Model file for the job. Use its own axes, mm. A direction names the side the tool comes from. Round coordinates to 2 decimals unless told otherwise and drop trailing zeros. Loops run counter-clockwise (first coordinate to the right, second up) from the corner with the lowest first, then second, coordinate; pieces in that order, holes last. Notation, with made-up numbers: M -24.5,31.5 L 13.5,31.5 A17 cw 13.5,38.5 Z; hole C 69.25,-5 d4. An arc over 180 degrees is marked long. Use a Markdown table: item, result. Add a question column.
Q1. Pin check, flat tips, straight feed: pin 1 (1.5 mm diameter, centred on x = 49.5, y = 1, fed in from +Z); pin 2 (1 mm diameter, centred on y = 1.5, z = 16, fed in from +X); pin 3 (3.5 mm diameter, centred on x = 12.5, z = 15, fed in from +Y). Stop position of each tip, or through.
Q2. Cut at C-C (x = 61). Give the cut face in (y, z).
Q3. Mould opens along Z. For faces 1 (the face through (47, 1, 7.5)), 2 (the face through (12.59, 1.48, 17.1)), 3 (the face through (-1, 3, 4)), 4 (the face through (-1, 1, -7.5)) say: +Z half, -Z half, draft (parallel to the pull), parting line (faces both ways), or undercut.
Q4. Probe line 1 (X direction, y = 1.4, z = 0); line 2 (X direction, y = 1.9, z = 15.25); line 3 (Z direction, x = 58, y = 2.1). List the from-to ranges inside material, lowest first. Write a range as from..to.
Q5. Cut at B-B (x = 42.5). Give the cut face in (y, z).
Q6. Tool access for faces 5 (the face through (-46, 1, 7.5)), 6 (the face through (-43.92, 1.48, 0.74)): list every direction of +Z, -Z, +X, -X, +Y, -Y with a clear straight run to the whole face (end or side of a thin tool).
Q7. Cut at A-A (y = 0.5). Give the cut face in (x, z).
Q8. Cut at D-D (z = 10.5). Give the cut face in (x, y), plus the area to 3 significant figures.
from build123d import *

# Parameters (mm, degrees)
SKETCH_1_R          = 1.6
SKETCH_1_R_2        = 2.1
EXTRUDE_1_DEPTH     = 3
SKETCH_3_W          = 40
SKETCH_3_H          = 3
EXTRUDE_3_DEPTH     = 15
SKETCH_2_R          = 2.1
CUT_EXTRUDE_1_DEPTH = 76.970388968
FILLET_START        = -1
FILLET_2_DEPTH      = 5
FILLET_2_2_DEPTH    = 3


with BuildPart() as part:
    # 草图1 → 凸台-拉伸1 (new body)
    with BuildSketch(Plane(origin=(0, 0, 0), x_dir=(1, 0, 0), z_dir=(0, 1, 0))):
        with BuildLine():
            Line((-65, 7.5), (65, 7.5))
            ThreePointArc((65, 7.5), (72.5, 0), (65, -7.5))
            Line((65, -7.5), (-65, -7.5))
            ThreePointArc((-65, -7.5), (-72.5, 0), (-65, 7.5))
        make_face()
        with Locations(Location((-42.5, 0, 0), (0, 0, 270))):
            Circle(SKETCH_1_R, mode=Mode.SUBTRACT)
        with Locations(Location((-65, 0, 0), (0, 0, 270))):
            Circle(SKETCH_1_R_2, mode=Mode.SUBTRACT)
        with Locations(Location((65, 0, 0), (0, 0, 270))):
            Circle(SKETCH_1_R_2, mode=Mode.SUBTRACT)
        with Locations(Location((42.5, 0, 0), (0, 0, 270))):
            Circle(SKETCH_1_R, mode=Mode.SUBTRACT)
    extrude(amount=EXTRUDE_1_DEPTH)

    # 草图3 → 凸台-拉伸3 (add)
    with BuildSketch(Plane.XY.offset(7.5)):
        with Locations((0, 1.5)):
            Rectangle(SKETCH_3_W, SKETCH_3_H)
    extrude(amount=EXTRUDE_3_DEPTH)

    # 草图2 → 切除-拉伸1 (cut, through all)
    with BuildSketch(Plane.XZ):
        with Locations(Location((-12.5, 15, 0), (0, 0, 270))):
            Circle(SKETCH_2_R)
        with Locations(Location((12.5, 15, 0), (0, 0, 270))):
            Circle(SKETCH_2_R)
    extrude(amount=-CUT_EXTRUDE_1_DEPTH, mode=Mode.SUBTRACT)

    # 圆角2: read off the stored shape, not the designer's step
    # 圆角2 outline → 圆角2 (cut)
    with BuildSketch(Plane(origin=(0, 0, 0), x_dir=(1, 0, 0), z_dir=(0, 1, 0)).offset(FILLET_START)):
        with BuildLine():
            ThreePointArc((20, -15), (17.803300859, -20.303300859), (12.5, -22.5))
            Line((12.5, -22.5), (20, -22.5))
            Line((20, -22.5), (20, -15))
        make_face()
        with BuildLine():
            Line((-20, -22.5), (-12.5, -22.5))
            ThreePointArc((-12.5, -22.5), (-17.803300859, -20.303300859), (-20, -15))
            Line((-20, -15), (-20, -22.5))
        make_face()
    extrude(amount=FILLET_2_DEPTH, mode=Mode.SUBTRACT)

    # Fillet 2 2 outline → Fillet 2 2 (add)
    with BuildSketch(Plane(origin=(0, 0, 0), x_dir=(1, 0, 0), z_dir=(0, 1, 0))):
        with BuildLine():
            Line((20, -7.5), (20, -15))
            ThreePointArc((20, -15), (22.196699141, -9.696699141), (27.5, -7.5))
            Line((27.5, -7.5), (20, -7.5))
        make_face()
        with BuildLine():
            ThreePointArc((-27.5, -7.5), (-22.196699141, -9.696699141), (-20, -15))
            Line((-20, -15), (-20, -7.5))
            Line((-20, -7.5), (-27.5, -7.5))
        make_face()
    extrude(amount=FILLET_2_2_DEPTH)


solid = part.part
Checked values:
| question | item | result |
|---|---|---|
| 1 | pin 1 | stops at z = 7.5 |
| 1 | pin 2 | stops at x = 19.98 |
| 1 | pin 3 | passes through |
| 2 | outline | M 0,-7.5 L 3,-7.5 L 3,7.5 L 0,7.5 Z |
| 3 | face 1 | +Z half |
| 3 | face 2 | undercut |
| 3 | face 3 | draft |
| 3 | face 4 | -Z half |
| 4 | line 1 | x = -72.5..-67.1, -62.9..-44.1, -40.9..40.9, 44.1..62.9, 67.1..72.5 |
| 4 | line 2 | x = -20..-14.59, -10.41..10.41, 14.59..20 |
| 4 | line 3 | z = -7.5..7.5 |
| 5 | outline | M 0,-7.5 L 3,-7.5 L 3,-1.6 L 0,-1.6 Z; M 0,1.6 L 3,1.6 L 3,7.5 L 0,7.5 Z |
| 6 | face 5 | +Z, -X, +Y, -Y |
| 6 | face 6 | +Y, -Y |
| 7 | outline | M -65,-7.5 L 65,-7.5 A7.5 ccw 65,7.5 L 27.5,7.5 A7.5 cw 20,15 A7.5 ccw 12.5,22.5 L -12.5,22.5 A7.5 ccw -20,15 A7.5 cw -27.5,7.5 L -65,7.5 A7.5 ccw Z; hole C -65,0 d4.2; hole C -42.5,0 d3.2; hole C -12.5,15 d4.2; hole C 12.5,15 d4.2; hole C 42.5,0 d3.2; hole C 65,0 d4.2 |
| 8 | outline | M -21.5,0 L 21.5,0 L 21.5,3 L -21.5,3 Z |
| 8 | area | 129 mm^2 |
